from build123d import *

# Parameters (mm, degrees)
SKETCH_1_R      = 32.5
EXTRUDE_1_DEPTH = 36
SKETCH_2_R      = 38.5
EXTRUDE_2_DEPTH = 82
SKETCH_3_R      = 41
EXTRUDE_3_DEPTH = 12
SKETCH_4_R      = 35
EXTRUDE_4_DEPTH = 76
SKETCH_5_R      = 32.5
EXTRUDE_5_DEPTH = 64
SKETCH_6_R      = 31
EXTRUDE_6_DEPTH = 50
SKETCH_7_R      = 27.5
EXTRUDE_7_DEPTH = 82
FILLET_1_R      = 2
FILLET_2_R      = 1.6
CHAMFER_1_SIZE  = 2


with BuildPart() as part:
    # 草图1 → 凸台-拉伸1 (new body)
    with BuildSketch(Plane.XY):
        Circle(SKETCH_1_R)
    extrude(amount=EXTRUDE_1_DEPTH)

    # 草图2 → 凸台-拉伸2 (add)
    with BuildSketch(Plane.XY.offset(36)):
        Circle(SKETCH_2_R)
    extrude(amount=EXTRUDE_2_DEPTH)

    # 草图3 → 凸台-拉伸3 (add)
    with BuildSketch(Plane.XY.offset(118)):
        Circle(SKETCH_3_R)
    extrude(amount=EXTRUDE_3_DEPTH)

    # 草图4 → 凸台-拉伸4 (add)
    with BuildSketch(Plane.XY.offset(130)):
        Circle(SKETCH_4_R)
    extrude(amount=EXTRUDE_4_DEPTH)

    # 草图5 → 凸台-拉伸5 (add)
    with BuildSketch(Plane.XY.offset(206)):
        Circle(SKETCH_5_R)
    extrude(amount=EXTRUDE_5_DEPTH)

    # 草图6 → 凸台-拉伸6 (add)
    with BuildSketch(Plane.XY.offset(270)):
        Circle(SKETCH_6_R)
    extrude(amount=EXTRUDE_6_DEPTH)

    # 草图7 → 凸台-拉伸7 (add)
    with BuildSketch(Plane.XY.offset(320)):
        Circle(SKETCH_7_R)
    extrude(amount=EXTRUDE_7_DEPTH)

    # 圆角1
    fillet_1_edges = [part.edges().sort_by_distance(p)[0] for p in [
        (-35, 0, 130),
        (-32.5, 0, 206),
    ]]
    fillet(fillet_1_edges, radius=FILLET_1_R)

    # 圆角2
    # the kernel refuses this fillet: 1.6 mm, written as the material it adds along each edge
    with BuildSketch(Plane(origin=(0, 0, 270), x_dir=(1, 0, 0), z_dir=(0, -1, 0))) as fillet_2_piece_1:
        with BuildLine():
            CenterArc((32.6, 1.596871942), FILLET_2_R, 180, 86.416678302)
            Line((31, 1.596871942), (30.968, 1.596871942))
            Line((30.968, 1.596871942), (30.968, 0))
            Line((30.968, 0), (31, -0.032))
            ThreePointArc((31, -0.032), (31.75, -0.032), (32.498, -0.031937439))
            Line((32.498, -0.031937439), (32.5, 0))
        make_face()
    revolve(axis=Axis((0, 0, 270), (0, 0, 1)))
    with BuildSketch(Plane(origin=(0, 0, 320), x_dir=(1, 0, 0), z_dir=(0, -1, 0))) as fillet_2_piece_2:
        with BuildLine():
            CenterArc((27.5 + FILLET_2_R, FILLET_2_R), FILLET_2_R, 180, 90)
            Line((27.5, FILLET_2_R), (27.5 - FILLET_2_R * 0.02, FILLET_2_R))
            Line((27.5 - FILLET_2_R * 0.02, FILLET_2_R), (27.5 - FILLET_2_R * 0.02, -FILLET_2_R * 0.02))
            Line((27.5 - FILLET_2_R * 0.02, -FILLET_2_R * 0.02), (27.5 + FILLET_2_R, -FILLET_2_R * 0.02))
            Line((27.5 + FILLET_2_R, -FILLET_2_R * 0.02), (27.5 + FILLET_2_R, 0))
        make_face()
    revolve(axis=Axis((0, 0, 320), (0, 0, 1)))

    # 倒角1
    chamfer_1_edges = [part.edges().sort_by_distance(p)[0] for p in [
        (-32.5, 0, 0),
        (-27.5, 0, 402),
    ]]
    chamfer(chamfer_1_edges, length=CHAMFER_1_SIZE)


solid = part.part
Model file for the job. Use its own axes, mm. A direction names the side the tool comes from. Give positions to 0.01 mm unless a question says otherwise; leave off trailing zeros. Order: outer loops, then holes, each group sorted by start corner. A loop starts at its lowest first (then second) coordinate and runs counter-clockwise, first axis right, second up. Notation, with made-up numbers: (70.5, -10.5) - (76.5, -10.5) arc R19 cw to (76.5, 8.5) - close; hole circle Ø9 at (8, -39.5). An arc over 180 degrees is marked (long way). Write item = value, one per line. Start each with the question number.
1. Cut at B-B, the plane z = 314. List the corners of the cut face in (x, y), and give its area (3 significant figures).
2. Drop flat-ended pins along their axis: P1, Ø1, axis at x = -11, y = 29, coming from the +Z side; P2, Ø8, axis at x = -3.5, z = 338.5, coming from the +Y side; P3, Ø3, axis at x = 24.5, z = 91.5, coming from the -Y side. Give the stop position or say it passes through.
3. Cut at A-A, the plane z = 230. List the corners of the cut face in (x, y), and give its area (3 significant figures).
4. Probe line 1 along Y through (x, z) = (2, 108); line 2 along Y through (x, z) = (0, 205); line 3 along Z through (x, y) = (26, -23). List the from-to ranges inside material, lowest first.
5. Which spindle directions (+Z, -Z, +X, -X, +Y, -Y) get a long thin tool onto all of the face, cutting with end or side? Do faces 1 (the flat face through (-26, -20, 36)), 2 (the flat face through (0, 0, 0)), 3 (the cylindrical face through (-5.961, -26.846, 360.251)). Say none if no direction does.
Taken from the geometry:
q1.outline = circle Ø62 at (0, 0)
q1.area = 3,020 mm²
q2.P1 = 320
q2.P2 = 27.5
q2.P3 = -30.87
q3.outline = circle Ø65 at (0, 0)
q3.area = 3,320 mm²
q4.line_1 = -38.45 to 38.45
q4.line_2 = -35 to 35
q4.line_3 = 36 to 206
q5.face_1 = -Z
q5.face_2 = -Z, +X, -X, +Y, -Y
q5.face_3 = +Z
